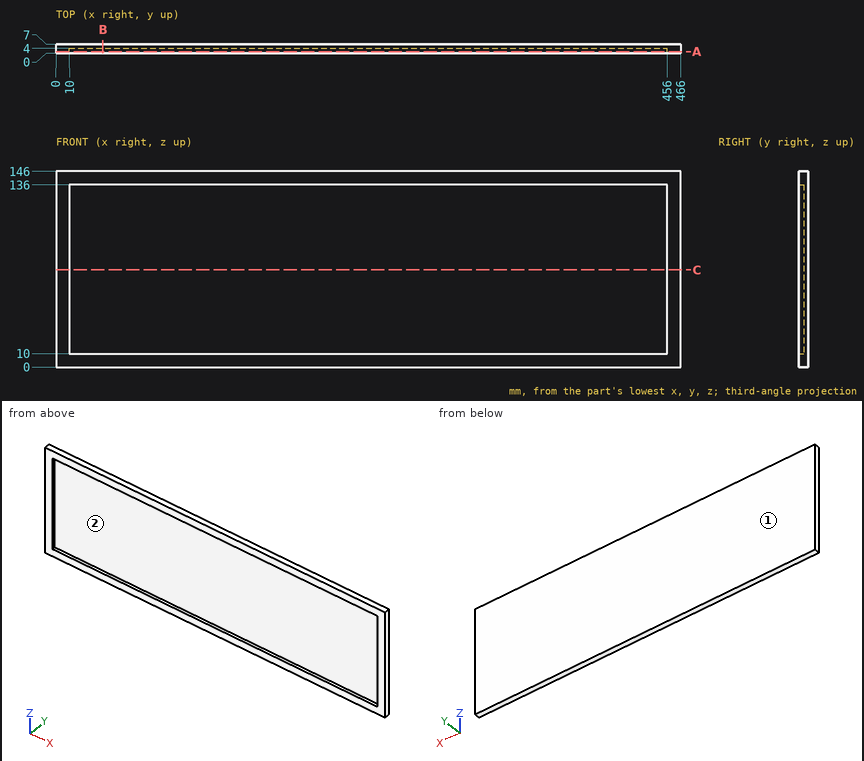
Job drawing, mm, ordinate dimensions from the low corner. One solid piece. Coordinates: 2 decimals unless noted, no trailing zeros. Write each loop counter-clockwise with the first axis right and the second up, starting at its lowest first coordinate (ties: lowest second). Pieces come first, ordered by that corner, then holes. Notation, with made-up numbers: M -30,2 L -2,2 A32 ccw -2,34 Z; hole C -28.5,62.5 d4. An arc over 180 degrees is marked long. Answer as a JSON object with one key per item and string values. Group by question number.
1) Wall check: line 1 (Z direction, x = 386.5, y = 1); line 2 (X direction, y = 1.5, z = 124); line 3 (Y direction, x = 287, z = 31). Give the ranges that are in metal, low to high. Write a range as from..to.
2) Mould opens along Z. For the marked faces 1 and 2 say: +Z half, -Z half, draft (parallel to the pull), parting line (faces both ways), or undercut.
3) Saw through at A-A (y = 1.25). Write the cut outline in (x, z), plus the area to 3 significant figures.
4) Saw through at B-B (x = 35). Write the cut outline in (y, z).
5) Pin check, flat tip, straight feed: pin 1 Ø6 at (x, z) = (254, 104) entering from -Y. Stop position of the tip, or through.
6) Saw through at C-C (z = 72.5). Write the cut outline in (x, y), plus the area to 3 significant figures.
Values follow:
{
 "1": {"line 1": "z = 0..10, 136..146", "line 2": "x = 0..10, 456..466", "line 3": "y = 4..7"},
 "2": {"face 1": "draft", "face 2": "undercut"},
 "3": {"outline": "M 0,0 L 466,0 L 466,146 L 0,146 Z; hole M 10,10 L 456,10 L 456,136 L 10,136 Z", "area": "11,800 mm2"},
 "4": {"outline": "M 0,0 L 7,0 L 7,146 L 0,146 L 0,136 L 4,136 L 4,10 L 0,10 Z"},
 "5": {"pin 1": "stops at y = 4"},
 "6": {"outline": "M 0,0 L 10,0 L 10,4 L 456,4 L 456,0 L 466,0 L 466,7 L 0,7 Z", "area": "1,480 mm2"}
}
